from build123d import *

# Parameters (mm, degrees)
CROQUIS1_W                                     = 25
CROQUIS1_H                                     = 50
SALIENTE_EXTRUIR1_DEPTH                        = 80
PERFORADOR_PARA_ROSCAR_PARA_MACHO_DE_ROS_D     = 4.2
PERFORADOR_PARA_ROSCAR_PARA_MACHO_DE_ROS_DEPTH = 11
PERFORADOR_PARA_ROSCAR_PARA_MACHO_DE_ROS_TIP   = 1.2618073
PERFORADOR_PARA_ROSCAR_PARA_MACHO_DE_2_D       = 4.2
PERFORADOR_PARA_ROSCAR_PARA_MACHO_DE_2_DEPTH   = 11
PERFORADOR_PARA_ROSCAR_PARA_MACHO_DE_2_TIP     = 1.2618073


with BuildPart() as part:
    # Croquis1 → Saliente-Extruir1 (new body)
    with BuildSketch(Plane.XY):
        with Locations((-19.131816286, 7.30620438)):
            Rectangle(CROQUIS1_W, CROQUIS1_H)
    extrude(amount=SALIENTE_EXTRUIR1_DEPTH)

    # Perforador para roscar para macho de ros
    with Locations(Plane(origin=(-21.631816286, 32.30620438, 40), x_dir=(0, 0, 1), z_dir=(0, 1, 0))):
        with Locations((0, 0)):
            Hole(PERFORADOR_PARA_ROSCAR_PARA_MACHO_DE_ROS_D / 2, depth=PERFORADOR_PARA_ROSCAR_PARA_MACHO_DE_ROS_DEPTH)
            with Locations((0, 0, -(PERFORADOR_PARA_ROSCAR_PARA_MACHO_DE_ROS_DEPTH + PERFORADOR_PARA_ROSCAR_PARA_MACHO_DE_ROS_TIP / 2))):  # 118° drill point
                Cone(0, PERFORADOR_PARA_ROSCAR_PARA_MACHO_DE_ROS_D / 2, PERFORADOR_PARA_ROSCAR_PARA_MACHO_DE_ROS_TIP, mode=Mode.SUBTRACT)

    # Perforador para roscar para macho de 2
    with Locations(Plane(origin=(-21.631816286, -17.69379562, 40), x_dir=(0, 0, -1), z_dir=(0, -1, 0))):
        with Locations((0, 0)):
            Hole(PERFORADOR_PARA_ROSCAR_PARA_MACHO_DE_2_D / 2, depth=PERFORADOR_PARA_ROSCAR_PARA_MACHO_DE_2_DEPTH)
            with Locations((0, 0, -(PERFORADOR_PARA_ROSCAR_PARA_MACHO_DE_2_DEPTH + PERFORADOR_PARA_ROSCAR_PARA_MACHO_DE_2_TIP / 2))):  # 118° drill point
                Cone(0, PERFORADOR_PARA_ROSCAR_PARA_MACHO_DE_2_D / 2, PERFORADOR_PARA_ROSCAR_PARA_MACHO_DE_2_TIP, mode=Mode.SUBTRACT)


solid = part.part
Could you check a few things on this model? Use its own coordinates, in mm. A direction names the side the tool comes from. Give positions to 0.01 mm unless a question says otherwise; leave off trailing zeros. Return JSON: item names as keys, results as strings.
1. Thinking about a two-plate mould opening in X: for faces 4 (the flat face through (-19, 8, 0)), 5 (the flat face through (-31.632, 7, 39)), 6 (the conical face through (-21.988, 20.264, 39.921)), which applies, pulls with the +X half, pulls with the -X half, needs draft (parallel to the pull), parting line crosses it, or undercut?
Answer list:
{"face 4": "needs draft", "face 5": "pulls with the -X half", "face 6": "undercut"}
2. On a 3-axis mill with a long thin cutter (end or side, diameter ignored), from which of +Z, -Z, +X, -X, +Y, -Y can I reach the whole of each face in a straight line? I mean faces 1 (the flat face through (-19, 32.306, 39)), 2 (the cylindrical face through (-21.539, -12.117, 37.902)), 3 (the cylindrical face through (-21.539, 26.729, 42.098)). Say none if no direction works.
Answer list:
{"face 1": "+Z, -Z, +X, -X, +Y", "face 2": "-Y", "face 3": "+Y"}
3. I need wall thicknesses on line 1 (X direction, y = -10.25, z = 40); line 2 (Z direction, x = -21, y = 22); line 3 (Z direction, x = -20, y = -14.5). Which ranges of each line are inside material? Lowest first, please. Write a range as from..to.
Answer list:
{"line 1": "x = -31.63..-23.73, -19.53..-6.63", "line 2": "z = 0..38, 42..80", "line 3": "z = 0..38.68, 41.32..80"}
